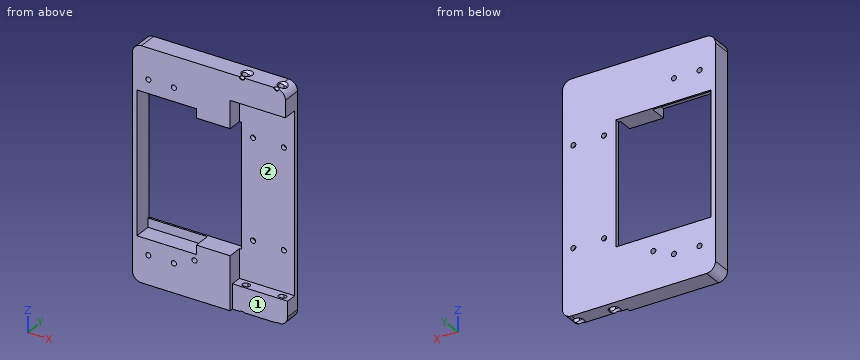
Autodesk Inventor part; units mm, degrees
ref_plane "Arbeitsebene3" through (-32.75, 5, -38) normal (0, 1, 0) x (0, 0, 1)
ref_plane "YZ Plane" through (0, 0, 0) normal (1, 0, 0) x (0, 1, 0)
ref_plane "XZ Plane" through (0, 0, 0) normal (0, 1, 0) x (-1, 0, 0)
sketch "Skizze1" plane through (0, 0, 0) normal (0, 1, 0) x (-1, 0, 0)
  line L0 (-37.25, -63.4) -> (37.25, -63.4)
  line L1 (42.25, -58.4) -> (42.25, 58.4)
  line L2 (37.25, 63.4) -> (-37.25, 63.4)
  line L3 (-42.25, 58.4) -> (-42.25, -58.4)
  line L4 (-42.25, -63.4) -> (42.25, 63.4) construction
  line L5 (42.25, -63.4) -> (-42.25, 63.4) construction
  arc A0 (42.25, 58.4) -> (37.25, 63.4) centre (37.25, 58.4) ccw
  arc A1 (-37.25, 63.4) -> (-42.25, 58.4) centre (-37.25, 58.4) ccw
  arc A2 (-42.25, -58.4) -> (-37.25, -63.4) centre (-37.25, -58.4) ccw
  arc A3 (37.25, -63.4) -> (42.25, -58.4) centre (37.25, -58.4) ccw
  point P0 (0, 0)
  dimension "d0" = 84.5
  dimension "d1" = 126.8
  dimension "d2" = 5
extrude "Extrusion1" add sketch "Skizze1" along normal blind 10.5
ref_plane "Arbeitsebene1" through (37.25, 0, 0) normal (0, 0, -1) x (-1, 0, 0)
ref_plane "Arbeitsebene2" through (0, 0, 58.4) normal (1, 0, 0) x (0, 0, -1)
sketch "Skizze2" plane through (0, 10.5, 0) normal (0, 1, 0) x (1, 0, 0)
  line L0 (-12.95, 38) -> (-38.75, 38)
  line L1 (-38.75, -38) -> (-12.95, -38)
  line L2 (-12.95, -38) -> (-12.95, -2.5)
  line L3 (-38.75, 38) -> (-38.75, -38)
  line L4 (-38.75, -38) -> (-12.95, -38)
  line L5 (-12.95, -38) -> (-12.95, 38)
  line L6 (-12.95, 38) -> (-38.75, 38)
  line L7 (-38.75, 38) -> (-38.75, -38)
  line L8 (-11.95, 39) -> (-11.95, -39)
  line L9 (-11.95, -39) -> (-39.75, -39)
  line L10 (-39.75, -39) -> (-39.75, 39)
  line L11 (-39.75, 39) -> (-11.95, 39)
  line L12 (-11.95, 39) -> (-6.95, 39)
  line L13 (-6.95, 39) -> (-6.95, -39)
  line L14 (-6.95, -39) -> (-11.95, -39)
  line L15 (-11.95, -39) -> (-11.95, 39)
  point P0 (0, 0)
  dimension "d5" = 1
  dimension "d64" = 5
extrude "Extrusion2" cut sketch "Skizze2" against normal through all contours L5 L2 L1 L3 L0 | L12 L13 L14 L8 | L8 L9 L10 L11
ref_plane "Arbeitsebene3" through (-32.75, 5, -38) normal (0, 1, 0) x (0, 0, 1)
sketch "Skizze3" plane through (0, 10.5, 0) normal (0, 1, 0) x (1, 0, 0)
  line L0 (-39.75, -39) -> (-39.75, 39)
  arc A0 (-37.25, 63.4) -> (-42.25, 58.4) centre (-37.25, 58.4) ccw
  line L1 (-42.25, 58.4) -> (-42.25, -58.4)
  arc A1 (-42.25, -58.4) -> (-37.25, -63.4) centre (-37.25, -58.4) ccw
  line L2 (-37.25, -63.4) -> (37.25, -63.4)
  arc A2 (37.25, -63.4) -> (42.25, -58.4) centre (37.25, -58.4) ccw
  line L3 (42.25, -58.4) -> (42.25, 58.4)
  arc A3 (42.25, 58.4) -> (37.25, 63.4) centre (37.25, 58.4) ccw
  line L4 (37.25, 63.4) -> (-37.25, 63.4)
  line L5 (-39.75, -39) -> (-39.75, 39)
  line L6 (-39.75, -39) -> (-6.95, -39)
  line L7 (-6.95, -39) -> (-6.95, -34)
  line L8 (-6.95, -34) -> (-39.75, -34)
  line L9 (-39.75, -34) -> (-39.75, -39)
  line L10 (-39.75, 39) -> (-6.95, 39)
  line L11 (-6.95, 39) -> (-6.95, 34)
  line L12 (-6.95, 34) -> (-39.75, 34)
  line L13 (-39.75, 34) -> (-39.75, 39)
  line L14 (-6.95, -39) -> (-39.75, -39)
  line L15 (-39.75, 39) -> (-6.95, 39)
  line L16 (-6.95, 39) -> (-6.95, -39)
  line L17 (-6.95, -39) -> (-6.95, 39)
  point P0 (0, 0)
  dimension "d8" = 32.8
  dimension "d9" = 5
  dimension "d10" = 5
extrude "Extrusion3" add sketch "Skizze3" against normal blind 1 contours L0 L8 L7 L6 | L0 L10 L11 L12
sketch "Skizze4" plane through (0, 0, 0) normal (0, -1, 0) x (1, 0, 0)
  line L0 (-39.75, -39) -> (-39.75, 39)
  arc A0 (-42.25, -58.4) -> (-37.25, -63.4) centre (-37.25, -58.4) ccw
  line L1 (37.25, -63.4) -> (-37.25, -63.4)
  arc A1 (37.25, -63.4) -> (42.25, -58.4) centre (37.25, -58.4) ccw
  line L2 (42.25, 58.4) -> (42.25, -58.4)
  arc A2 (42.25, 58.4) -> (37.25, 63.4) centre (37.25, 58.4) ccw
  line L3 (-37.25, 63.4) -> (37.25, 63.4)
  arc A3 (-37.25, 63.4) -> (-42.25, 58.4) centre (-37.25, 58.4) ccw
  line L4 (-42.25, -58.4) -> (-42.25, 58.4)
  line L5 (-11.95, -34) -> (-11.95, 34)
  line L6 (-11.95, 34) -> (12.75, 34)
  line L7 (12.75, 34) -> (12.75, -34)
  line L8 (12.75, -34) -> (-11.95, -34)
  line L9 (-11.95, -34) -> (-11.95, 34)
  line L10 (-2.45, 7.5) -> (-2.45, -8)
  line L11 (12.75, -34.1) -> (12.75, -39.1)
  line L12 (-39.75, 39) -> (-6.95, 39)
  line L13 (-6.95, 39) -> (-6.95, -39)
  line L14 (-6.95, -39) -> (-39.75, -39)
  point P0 (0, 0)
  dimension "d44" = 0
extrude "Extrusion4" cut sketch "Skizze4" against normal through all contours L13 L6 L7 L8 | L8 L5 L6 L13
sketch "Skizze5" plane through (0, 0, 0) normal (0, -1, 0) x (1, 0, 0)
  arc A0 (-42.25, -58.4) -> (-37.25, -63.4) centre (-37.25, -58.4) ccw
  line L0 (37.25, -63.4) -> (-37.25, -63.4)
  arc A1 (37.25, -63.4) -> (42.25, -58.4) centre (37.25, -58.4) ccw
  line L1 (42.25, 58.4) -> (42.25, -58.4)
  arc A2 (42.25, 58.4) -> (37.25, 63.4) centre (37.25, 58.4) ccw
  line L2 (-37.25, 63.4) -> (37.25, 63.4)
  arc A3 (-37.25, 63.4) -> (-42.25, 58.4) centre (-37.25, 58.4) ccw
  line L3 (-42.25, -58.4) -> (-42.25, 58.4)
  line L4 (-6.95, 34) -> (12.75, 34)
  line L5 (12.75, 34) -> (12.75, -34)
  line L6 (12.75, -34) -> (-6.95, -34)
  line L7 (-39.75, -39) -> (-39.75, 39)
  line L8 (-6.95, -34) -> (-6.95, -39)
  line L9 (-6.95, -39) -> (-39.75, -39)
  line L10 (-39.75, 39) -> (-6.95, 39)
  line L11 (-6.95, 39) -> (-6.95, 34)
  circle A4 centre (-33.4798, 46.5) radius 1.4
  circle A5 centre (-33.4798, -47.5) radius 1.4
  circle A6 centre (-19.35, -47.5) radius 1.4
  circle A7 centre (-19.35, 46.5) radius 1.4
  circle A8 centre (-7.95, -42.5) radius 1.4
  point P0 (0, 0)
extrude "Extrusion5" cut sketch "Skizze5" against normal through all contours A4 | A5 | A6 | A7 | A8
sketch "Skizze9" plane through (0, 10.5, 0) normal (0, -1, 0) x (1, 0, 0)
  arc A0 (-42.25, -58.4) -> (-37.25, -63.4) centre (-37.25, -58.4) ccw
  line L0 (37.25, -63.4) -> (-37.25, -63.4)
  arc A1 (37.25, -63.4) -> (42.25, -58.4) centre (37.25, -58.4) ccw
  line L1 (42.25, 58.4) -> (42.25, -58.4)
  arc A2 (42.25, 58.4) -> (37.25, 63.4) centre (37.25, 58.4) ccw
  line L2 (-37.25, 63.4) -> (37.25, 63.4)
  arc A3 (-37.25, 63.4) -> (-42.25, 58.4) centre (-37.25, 58.4) ccw
  line L3 (-42.25, -58.4) -> (-42.25, 58.4)
  line L4 (12.75, 34) -> (12.75, -34)
  line L5 (12.75, -34) -> (-6.95, -34)
  line L6 (-39.75, -39) -> (-39.75, 39)
  line L7 (-6.95, 34) -> (12.75, 34)
  line L8 (-39.75, 39) -> (-11.95, 39)
  line L9 (-39.75, 39) -> (-11.95, 39)
  line L10 (-11.95, 39) -> (-11.95, 34)
  line L11 (-11.95, 34) -> (-39.75, 34)
  line L12 (-39.75, 34) -> (-39.75, 39)
  line L13 (-11.95, -39) -> (-39.75, -39)
  line L14 (-39.75, -39) -> (-39.75, -34)
  line L15 (-11.95, -39) -> (-39.75, -39)
  line L16 (-39.75, -39) -> (-39.75, -34)
  line L17 (-39.75, -34) -> (-11.95, -34)
  line L18 (-11.95, -34) -> (-11.95, -39)
  line L19 (-39.75, -39) -> (-9.75, -39)
  line L20 (-9.75, -39) -> (-9.75, 39)
  line L21 (-9.75, 39) -> (-39.75, 39)
  line L22 (-39.75, 39) -> (-39.75, -39)
  line L23 (-6.95, -34) -> (-6.95, -39)
  line L24 (-6.95, -39) -> (-39.75, -39)
  line L25 (-39.75, 39) -> (-6.95, 39)
  line L26 (-6.95, 39) -> (-6.95, 34)
  point P0 (0, 0)
  dimension "d63" = 30
extrude "Extrusion8" add sketch "Skizze9" along normal blind 1 contours L13 L6 L17 L18
sketch "Skizze10" plane through (0, 10.5, 0) normal (0, 1, 0) x (1, 0, 0)
  circle A0 centre (36.25, -27.6) radius 1.7
  circle A1 centre (19.25, -27.6) radius 1.7
  circle A2 centre (36.25, 27.4) radius 3.25
  circle A3 centre (19.25, 27.4) radius 3.25
  point P0 (0, 0)
  point P1 (19.25, -37.4)
  point P2 (19.25, 17.6)
  point P3 (36.25, -37.4)
  point P4 (36.25, 17.6)
hole "Bohrung2" at (19.25, 10.5, 27.6) at (36.25, 10.5, 27.6) at (19.25, 10.5, -27.4) at (36.25, 10.5, -27.4) direction (0, -1, 0) diameter 2.8 end through all
sketch "Skizze11" plane through (42.25, 0, 58.4) normal (1, 0, 0) x (0, 0, -1)
  line L0 (114.8, 1.25) -> (128.8, 1.25)
  line L1 (107.8, 1.4) -> (114.8, 1.4)
  line L2 (107.8, -25.5) -> (107.8, 7.5)
  line L3 (9.8, -20.5) -> (9.8, 7.5)
  line L4 (107.8, 7.5) -> (9.8, 7.5)
  line L5 (9.8, 7.5) -> (9.8, -20.5)
  line L6 (9.8, -20.5) -> (107.8, -20.5)
  line L7 (107.8, -20.5) -> (107.8, 7.5)
  line L8 (107.8, 1.4) -> (139.6262, 1.4)
  line L9 (139.6262, 1.4) -> (139.6262, -24.4892)
  line L10 (139.6262, -24.4892) -> (107.8, -24.4892)
  line L11 (107.8, -24.4892) -> (107.8, 1.4)
  line L12 (108.3, -21) -> (9.3, -21)
  line L13 (9.3, -21) -> (9.3, 8)
  line L14 (9.3, 8) -> (108.3, 8)
  line L15 (108.3, 8) -> (108.3, -21)
  line L16 (107.3, -24.9892) -> (140.1262, -24.9892)
  line L17 (140.1262, -24.9892) -> (140.1262, 1.9)
  line L18 (140.1262, 1.9) -> (107.3, 1.9)
  line L19 (107.3, 1.9) -> (107.3, -24.9892)
  point P0 (58.4, 0)
  point P1 (107.3, -21)
  point P2 (108.3, 1.9)
  dimension "d45" = 0.5
  dimension "d46" = 0.5
extrude "Extrusion9" cut sketch "Skizze11" against normal blind 30.5
sketch "Skizze12" plane through (-37.25, 0, 63.4) normal (0, 0, 1) x (1, 0, 0)
  circle A0 centre (75.5, 4.5) radius 2.75
  circle A1 centre (55.5, 4.5) radius 1.45
  circle A2 centre (75.5, 4.5) radius 1.45
  circle A3 centre (55.5, 4.5) radius 1.45
  point P0 (37.25, 0)
hole "Bohrung3" at (38.25, 4.5, 63.4) at (18.25, 4.5, 63.4) direction (0, 0, -1) diameter 3.2 end through all countersink diameter 6 countersink angle 90
sketch "Skizze13" plane through (37.25, 10.5, -63.4) normal (0, 0, -1) x (-1, 0, 0)
  circle A0 centre (0, -6) radius 2.75
  circle A1 centre (20, -6) radius 2.75
  point P0 (37.25, -10.5)
hole "Bohrung4" at (37.25, 4.5, -63.4) at (17.25, 4.5, -63.4) direction (0, 0, 1) diameter 3.2 end through all countersink diameter 6 countersink angle 90
sketch "Skizze14" plane through (0, 0, 0) normal (0, -1, 0) x (1, 0, 0)
  line L0 (19.85, 62) -> (16.65, 62)
  line L1 (39.85, 62) -> (36.65, 62)
  line L2 (16.15, -62.5) -> (19.35, -62.5)
  line L3 (36.15, -62.5) -> (39.35, -62.5)
  line L4 (35.7533, -63.4) -> (18.7467, -63.4)
  arc A0 (38.4354, -63.2575) -> (42.25, -58.4) centre (37.25, -58.4) ccw
  line L5 (42.25, -49.9) -> (42.25, -58.4)
  line L6 (42.25, -49.9) -> (11.75, -49.9)
  line L7 (11.75, -49.9) -> (11.75, -63.4)
  line L8 (-37.25, 63.4) -> (37.25, 63.4)
  line L9 (37.25, -63.4) -> (-37.25, -63.4)
  line L10 (15.7533, -63.4) -> (11.75, -63.4)
  point P0 (0, 0)
  point P1 (16.2533, -63.9)
  point P2 (19.2467, -63.9)
  point P3 (36.2533, -63.9)
  point P4 (18.25, 63.4)
  point P5 (17.75, -63.9)
  point P6 (-37.25, -63.4)
hole "Bohrung5" at (18.25, 0, 63.4) at (37.25, 0, 63.4) at (17.75, 0, -63.9) at (37.25, 0, -63.4) direction (0, 1, 0) diameter 2.8 depth 0.5 tip angle 118
properties part number "TIRFImager_base_50mm_NEMA11_v3"
Input: part model. Units: mm. Frame: model coordinates. Face numbers are marked on the shaded views. Give positions to 0.01 mm unless a question says otherwise; leave off trailing zeros. Write each loop counter-clockwise with the first axis right and the second up, starting at its lowest first coordinate (ties: lowest second). Pieces come first, ordered by that corner, then holes. Notation, with made-up numbers: (71, -29.5) -> (93, -29.5) arc R5 ccw to (93, -25.5) -> close; hole circle Ø11 at (12, 63.25). An arc over 180 degrees is marked (long way). Use one line per item in the form item = value. Start each with the question number.
1) Section query C-C on z = -24.5. Return the cut outline in (x, y), then the cut area to 3 significant figures.
2) Section query B-B on x = 9.5. Return the cut outline in (y, z), then the cut area to 3 significant figures.
3) Pin query (flat end, axial travel): pin 1 (3.5 mm diameter, centred on x = 38.25, y = 4.5, fed in from -Z); pin 2 (9 mm diameter, centred on x = 34, z = -1, fed in from -Y); pin 3 (3 mm diameter, centred on y = 1.5, z = 12.5, fed in from +X). Return the tip coordinate at first contact, or that it passes through.
4) Section query D-D on z = 46.5. Return the cut outline in (x, y), then the cut area to 3 significant figures.
5) Ray query, probe 1 along Z at (x, y) = (19.25, 9.05); probe 2 along Z at (x, y) = (-33.5, 1.75); probe 3 along X at (y, z) = (4.5, 56.5). Return the intervals inside material, ascending. Write a range as from..to.
6) Section query A-A on z = 27.6. Return the cut outline in (x, y).
7) Draft query along Z for the marked faces 1 and 2. Return one class per face: pulls with the +Z half, pulls with the -Z half, needs draft (parallel to the pull), parting line crosses it, or undercut.
Outcome:
q1.outline = (-42.25, 0) -> (-39.75, 0) -> (-39.75, 10.5) -> (-42.25, 10.5) -> close; (12.75, 8) -> (42.25, 8) -> (42.25, 10.5) -> (12.75, 10.5) -> close
q1.area = 100 mm^2
q2.outline = (0, -63.4) -> (10.5, -63.4) -> (10.5, -34) -> (0, -34) -> close; (0, 34) -> (10.5, 34) -> (10.5, 63.4) -> (0, 63.4) -> close
q2.area = 617 mm^2
q3.pin_1 = -62.92
q3.pin_2 = 8
q3.pin_3 = -39.75
q4.outline = (-42.25, 0) -> (-34.88, 0) -> (-34.88, 10.5) -> (-42.25, 10.5) -> close; (-32.08, 0) -> (-20.75, 0) -> (-20.75, 10.5) -> (-32.08, 10.5) -> close; (-17.95, 0) -> (11.75, 0) -> (11.75, 8) -> (42.25, 8) -> (42.25, 10.5) -> (-17.95, 10.5) -> close
q4.area = 584 mm^2
q5.probe_1 = -63.4..-28.8, -26..26.2, 29..63.4
q5.probe_2 = -63.4..-48.9, -46.1..-39, 39..45.1, 47.9..63.4
q5.probe_3 = -42.25..15.65, 19.85..35.65, 39.85..42.25
q6.outline = (-42.25, 0) -> (-39.75, 0) -> (-39.75, 10.5) -> (-42.25, 10.5) -> close; (12.75, 8) -> (17.85, 8) -> (17.85, 10.5) -> (12.75, 10.5) -> close; (20.65, 8) -> (34.85, 8) -> (34.85, 10.5) -> (20.65, 10.5) -> close; (37.65, 8) -> (42.25, 8) -> (42.25, 10.5) -> (37.65, 10.5) -> close
q7.face_1 = needs draft
q7.face_2 = undercut
